```python
from build123d import *

# Parameters (mm, degrees)
F0_R     = 63.5
F1_DEPTH = 76.2
F6_R     = 5.08
F7_SIZE  = 5.08


# Not quite as in the source:
# - the program builds the solid bodies; features that only make, move or delete a surface that nothing else refers to are left out


with BuildPart() as f1:
    # F0 (on Front) → F1 (new body)
    with BuildSketch(Plane.XZ):
        Circle(F0_R)
    extrude(amount=F1_DEPTH)

    # F6
    f6_edges = [f1.edges().sort_by_distance(p)[0] for p in [
        (-63.5, -76.2, 0),
    ]]
    fillet(f6_edges, radius=F6_R)

    # F7
    f7_edges = [f1.edges().sort_by_distance(p)[0] for p in [
        (-63.5, 0, 0),
    ]]
    chamfer(f7_edges, length=F7_SIZE)


solid = f1.part
```
Verification items for the finished model (mm, model axes). Round coordinates to 2 decimals unless told otherwise and drop trailing zeros. Order: outer loops, then holes, each group sorted by start corner. A loop starts at its lowest first (then second) coordinate and runs counter-clockwise, first axis right, second up. Notation, with made-up numbers: (66, 13) -> (75, 13) arc R30 cw to (75, 46) -> close; hole circle Ø8 at (76.25, -9.5). An arc over 180 degrees is marked (long way). Put each result on its own line as item: value. Start each with the question number.
(1) Section check A-A (y = -58). Enter the section's corners in (x, z), then the cut area to 3 significant figures.
(2) Depth check by flat-ended pin: pin 1 Ø2 at (x, y) = (-27.5, -33) entering from +Z; pin 2 Ø12 at (x, y) = (46.5, -53.5) entering from +Z; pin 3 Ø10 at (x, y) = (-1, -25) entering from +Z. Enter the tip coordinate at first touch or a pass-through.
(3) Draft check along Y on faces 1 (the face through (-1, -76.2, 1)), 2 (the face through (-1, 0, 1)), 3 (the face through (-13.77, -37.64, -61.99)). Enter one of: +Y half, -Y half, draft (parallel to the pull), parting line (faces both ways), or undercut.
(4) Material ranges on line 1 along Z through (x, y) = (2, -71); line 2 along X through (y, z) = (-34, -10.5); line 3 along Z through (x, y) = (-12, -40), recorded low to high.
Completed:
1. outline: circle Ø127 at (0, 0)
1. area: 12,700 mm2
2. pin 1: stops at z = 57.71
2. pin 2: stops at z = 48.91
2. pin 3: stops at z = 63.5
3. face 1: -Y half
3. face 2: +Y half
3. face 3: draft
4. line 1: z = -63.47 to 63.47
4. line 2: x = -62.63 to 62.63
4. line 3: z = -62.36 to 62.36
